Geometry check sheet. Reference: the model listing, model coordinates, mm. Face numbers are marked on the shaded views. Coordinates: 2 decimals unless noted, no trailing zeros. Write each loop counter-clockwise with the first axis right and the second up, starting at its lowest first coordinate (ties: lowest second). Pieces come first, ordered by that corner, then holes. Notation, with made-up numbers: M -26.75,8.5 L 3.25,8.5 A19 cw 3.25,41.5 Z; hole C -12.5,30.5 d8. An arc over 180 degrees is marked long. Write each question's results on one line, items separated by ' | '.
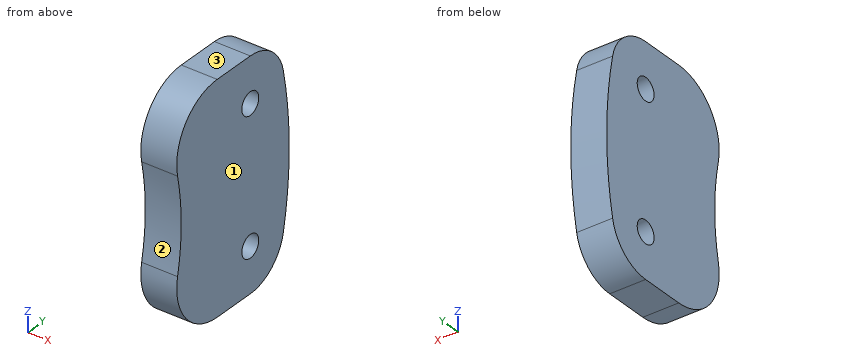
```python
from build123d import *

# Parameters (mm, degrees)
SKETCH2_R             = 3
BOSS_EXTRUDE1_DEPTH   = 4
FILLET1_R             = 6
M3X0_5_TAPPED_HOLE1_D = 2.5


with BuildPart() as part:
    # Sketch2 → Boss-Extrude1 (new body)
    # profile 1 of 2: a face of its own
    with BuildSketch(Plane(origin=(0, 0, 0), x_dir=(0, 0, -1), z_dir=(1, 0, 0))):
        with BuildLine():
            Line((12.5, 9.80532533), (12.5, -3.628540469))
            ThreePointArc((12.5, -3.628540469), (0, -0.426566699), (-12.5, -3.628540469))
            Line((-12.5, -3.628540469), (-12.5, 9.80532533))
            ThreePointArc((-12.5, 9.80532533), (-11.377342361, 12.962256786), (-8.513513514, 14.701526956))
            ThreePointArc((-8.513513514, 14.701526956), (0, 15.573433301), (8.513513514, 14.701526956))
            ThreePointArc((8.513513514, 14.701526956), (11.377342361, 12.962256786), (12.5, 9.80532533))
        make_face()
        with Locations((0, 10.573433301)):
            Circle(SKETCH2_R, mode=Mode.SUBTRACT)
    # profile 2 of 2: a face of its own
    with BuildSketch(Plane(origin=(0, 0, 0), x_dir=(0, 0, -1), z_dir=(1, 0, 0))):
        with Locations((0, 10.573433301)):
            Circle(SKETCH2_R)
    extrude(amount=BOSS_EXTRUDE1_DEPTH)

    # Fillet1
    fillet1_edges = [part.edges().sort_by_distance(p)[0] for p in [
        (2, -3.628540469, -12.5),
        (2, -3.628540469, 12.5),
    ]]
    fillet(fillet1_edges, radius=FILLET1_R)

    # M3x0.5 Tapped Hole1 (through all)
    with Locations(Plane.ZY):
        with Locations((-7.5, 9.80532533), (7.5, 9.80532533)):
            Hole(M3X0_5_TAPPED_HOLE1_D / 2)


solid = part.part
```
Q1. Sectioned sample at D-D on z = -2.5. Record the cut outline in (x, y), and give its area (3 significant figures).
Geometry check:
outline: M 0,-0.55 L 4,-0.55 L 4,15.5 L 0,15.5 Z | area: 64.2 mm2
Q2. Scan lines: probe 1 along Z at (x, y) = (1.45, 10.5); probe 2 along Z at (x, y) = (1.7, 4.75); probe 3 along Y at (x, z) = (0.8, 7.5). Record each from-to range of solid material in increasing order.
Geometry check:
probe 1: z = -12.45 to -8.54, -6.46 to 6.46, 8.54 to 12.45 | probe 2: z = -12.5 to 12.5 | probe 3: y = -1.01 to 8.56, 11.06 to 14.9
Q3. Sectioned sample at C-C on y = 11.75. Record the cut outline in (x, z).
Geometry check:
outline: M 0,-12.11 L 4,-12.11 L 4,12.11 L 0,12.11 Z
Q4. Mould release check, pull along Z, two halves, no side actions. Record for the marked faces 1, 2 and 3: pulls with the +Z half, pulls with the -Z half, needs draft (parallel to the pull), parting line crosses it, or undercut.
Geometry check:
face 1: needs draft | face 2: undercut | face 3: pulls with the +Z half
Q5. Depth check by flat-ended pin: P1, Ø1, axis at x = 1.5, z = 9.5, coming from the -Y side; P2, Ø4, axis at y = 9.81, z = -7.5, coming from the -X side; P3, Ø1, axis at x = 2, z = 8.5, coming from the +Y side. Enter the tip coordinate at first touch or a pass-through.
Geometry check:
P1: stops at y = -0.55 | P2: stops at x = 0 | P3: stops at y = 14.8
Q6. Sectioned sample at A-A on x = 1.2. Record the cut outline in (y, z), and give its area (3 significant figures).
Geometry check:
outline: M -0.97,-5.28 A6 ccw 4.91,-12.5 L 9.81,-12.5 A5 ccw 14.7,-8.51 A42 ccw 14.7,8.51 A5 ccw 9.81,12.5 L 4.91,12.5 A6 ccw -0.97,5.28 A26 cw Z; hole C 9.81,-7.5 d2.5; hole C 9.81,7.5 d2.5 | area: 364 mm2
Q7. Sectioned sample at B-B on z = 7.5. Record the cut outline in (x, y), and give its area (3 significant figures).
Geometry check:
outline: M 0,-1.01 L 4,-1.01 L 4,8.56 L 0,8.56 Z; M 0,11.06 L 4,11.06 L 4,14.9 L 0,14.9 Z | area: 53.6 mm2
